Part model, mm, in its own coordinate system. A direction names the side the tool comes from. Coordinates: 2 decimals unless noted, no trailing zeros. Loops run counter-clockwise (first coordinate to the right, second up) from the corner with the lowest first, then second, coordinate; pieces in that order, holes last. Notation, with made-up numbers: M -24.5,71 L 2.5,71 A7 cw 2.5,79 Z; hole C 24,18 d6. An arc over 180 degrees is marked long. Use a Markdown table: item, result. Add a question column.
1) Band-saw the part on A-A (x = 23.5). List the corners of the cut face in (y, z).
2) Pull direction Z, two halves, no side cores. Call faces 1 (the flat face through (26, -1060, 75)), 2 (the flat face through (22, -1060, 0)), 3 (the flat face through (4, -2150, 40)): released by +Z, released by -Z, zero draft, split by the parting line, or undercut.
3) Band-saw the part on B-B (y = -1088). List the corners of the cut face in (x, z).
4) Pin check, flat tips, straight feed: pin 1 Ø5 at (y, z) = (-742, 33) entering from +X; pin 2 Ø2 at (y, z) = (-337, 26.5) entering from -X. Stop position of each tip, or through.
5) Tool access for faces 4 (the flat face through (5, -1060, 40)), 5 (the flat face through (4, 0, 40)): list every direction of +Z, -Z, +X, -X, +Y, -Y with a clear straight run to the whole face (end or side of a thin tool).
6) Wall check: probe 1 along Z at (x, y) = (19.5, -943.5); probe 2 along X at (y, z) = (-1750.5, 65); probe 3 along X at (y, z) = (-1277.5, 9). Give the ranges that are in metal, low to high. Write a range as from..to.
7) Band-saw the part on C-C (z = 31.5). List the corners of the cut face in (x, y), plus the area to 4 significant figures.
from build123d import *

# Parameters (mm, degrees)
F1_DEPTH = 2150


with BuildPart() as f1:
    # F0 (on Front) → F1 (new body)
    with BuildSketch(Plane.XZ):
        with BuildLine():
            Line((0, 80), (0, 0))
            Line((0, 0), (45, 0))
            Line((45, 0), (45, 3))
            ThreePointArc((45, 3), (44.414214, 4.414214), (43, 5))
            Line((43, 5), (10, 5))
            ThreePointArc((10, 5), (6.464466, 6.464466), (5, 10))
            Line((5, 10), (5, 70))
            ThreePointArc((5, 70), (6.464466, 73.535534), (10, 75))
            Line((10, 75), (43, 75))
            ThreePointArc((43, 75), (44.414214, 75.585786), (45, 77))
            Line((45, 77), (45, 80))
            Line((45, 80), (0, 80))
        make_face()
    extrude(amount=F1_DEPTH)


solid = f1.part
Entries:
| question | item | result |
|---|---|---|
| 1 | outline | M -2150,0 L 0,0 L 0,5 L -2150,5 Z; M -2150,75 L 0,75 L 0,80 L -2150,80 Z |
| 2 | face 1 | undercut |
| 2 | face 2 | released by -Z |
| 2 | face 3 | zero draft |
| 3 | outline | M 0,0 L 45,0 L 45,3 A2 ccw 43,5 L 10,5 A5 cw 5,10 L 5,70 A5 cw 10,75 L 43,75 A2 ccw 45,77 L 45,80 L 0,80 Z |
| 4 | pin 1 | x = 5 |
| 4 | pin 2 | x = 0 |
| 5 | face 4 | +X, +Y, -Y |
| 5 | face 5 | +Z, -Z, +X, -X, +Y |
| 6 | probe 1 | 0..5, 75..80 |
| 6 | probe 2 | 0..5 |
| 6 | probe 3 | 0..5.1 |
| 7 | outline | M 0,-2150 L 5,-2150 L 5,0 L 0,0 Z |
| 7 | area | 10,750 mm2 |
